Can you work these out from the model? Positions are in its coordinate system, mm. Round coordinates to 2 decimals unless told otherwise and drop trailing zeros. Order: outer loops, then holes, each group sorted by start corner. A loop starts at its lowest first (then second) coordinate and runs counter-clockwise, first axis right, second up. Notation, with made-up numbers: M 86,-31.5 L 121,-31.5 A21 ccw 121,-17.5 Z; hole C 12,13.25 d11. An arc over 180 degrees is marked long. Answer as CSV lines item,"result". Start each with the question number.
from build123d import *

# Parameters (mm, degrees)
FRONT_FLOOR_CLOSEOUT_DEPTH = 1


with BuildPart() as part:
    # Sketch1 → Front Floor Closeout (new body)
    with BuildSketch(Plane(origin=(0, 0, 0), x_dir=(1, 0, 0), z_dir=(0, 1, 0))):
        Polygon((-247.7, 0), (247.7, 0), (247.7, 12.02), (294.245, 888.034340907), (-294.245, 888.034340907), (-247.7, 12.02), align=None)
    extrude(amount=FRONT_FLOOR_CLOSEOUT_DEPTH)


solid = part.part
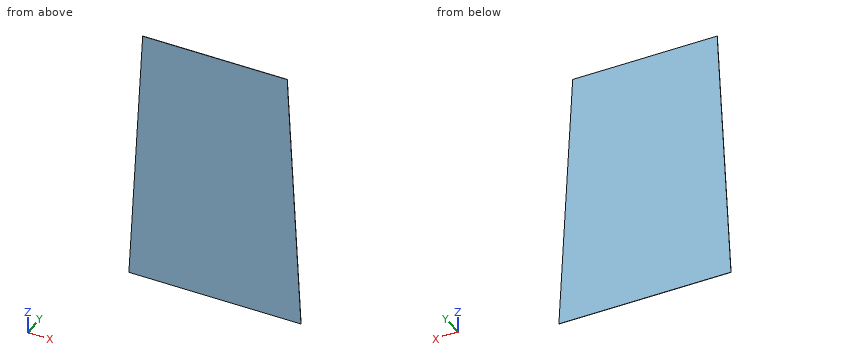
(1) I'm going to push a flat-ended pin straight in: P1, Ø0.5, axis at y = 0.5, z = -7.5, coming from the +X side. Where does the tip first touch, or does it pass through?
(2) I want a section at B-B on z = -739.5. Write out the boundary of the cut face in (x, y).
(3) If I drill on line 1 along X through (y, z) = (0.45, -770); line 2 along X through (y, z) = (0.75, -745), over which ranges is the centre line in solid material (lowest first)?
(4) I want a section at C-C on z = -458.5. Write out the boundary of the cut face in (x, y).
(5) I want a section at A-A on y = 0.7. Write out the boundary of the cut face in (x, z) (3 decimals).
From the geometry:
1,P1,"x = 247.7"
2,outline,"M -286.35,0 L 286.35,0 L 286.35,1 L -286.35,1 Z"
3,line 1,"-287.97 to 287.97"
3,line 2,"-286.65 to 286.65"
4,outline,"M -271.42,0 L 271.42,0 L 271.42,1 L -271.42,1 Z"
5,outline,"M -294.245,-888.034 L 294.245,-888.034 L 247.7,-12.02 L 247.7,0 L -247.7,0 L -247.7,-12.02 Z"
